from build123d import *

# Parameters (mm, degrees)
F0_R        = 15
F0_R_2      = 12
F1_DEPTH    = 1
F0_R_3      = 11.25
F2_DEPTH    = 7
F3_START    = 5
F1_FACE_R   = 15
F1_FACE_R_2 = 12
F3_DEPTH    = 1
F4_R        = 2


with BuildPart() as f1:
    # F0 (on Top) → F1 (new body)
    with BuildSketch(Plane.XY):
        Circle(F0_R)
        Circle(F0_R_2, mode=Mode.SUBTRACT)
    extrude(amount=F1_DEPTH)

    # F0 (on Top) → F2 (join)
    with BuildSketch(Plane.XY):
        Circle(F0_R_2)
        Circle(F0_R_3, mode=Mode.SUBTRACT)
    extrude(amount=F2_DEPTH)

    # F1_face (on face) → F3 (join)
    with BuildSketch(Plane.XY.offset(1).offset(F3_START)):
        Circle(F1_FACE_R)
        Circle(F1_FACE_R_2, mode=Mode.SUBTRACT)
    extrude(amount=F3_DEPTH)

    # F4
    f4_edges = [f1.edges().sort_by_distance(p)[0] for p in [
        (12, 0, 3.5),
        (-12, 0, 6),
        (-12, 0, 1),
    ]]
    fillet(f4_edges, radius=F4_R)


solid = f1.part
Check sheet for the modelled part. Datum: model origin and axes. Units: mm. Give positions to 0.01 mm unless a question says otherwise; leave off trailing zeros. Write each loop counter-clockwise with the first axis right and the second up, starting at its lowest first coordinate (ties: lowest second). Pieces come first, ordered by that corner, then holes. Notation, with made-up numbers: M 23,57 L 70,57 A20 cw 70,73 Z; hole C 41.25,-0.75 d8. An arc over 180 degrees is marked long. Use one line per item in the form item = value.
(1) Section check D-D on z = 5. Record the boundary of the cut face in (x, y), plus the area to 3 significant figures.
Answer block:
outline = C 0,0 d24.54; hole C 0,0 d22.5
area = 75.2 mm2
(2) Section check C-C on z = 2.5. Record the boundary of the cut face in (x, y), plus the area to 3 significant figures.
Answer block:
outline = C 0,0 d24.13; hole C 0,0 d22.5
area = 59.6 mm2
(3) Material ranges on line 1 along Y through (x, z) = (0, 3); line 2 along Z through (x, y) = (-11.5, -7.25); line 3 along X through (y, z) = (8.25, 5.75), recorded low to high.
Answer block:
line_1 = -12 to -11.25, 11.25 to 12
line_2 = 0 to 1.04, 5.96 to 7
line_3 = -10.09 to -7.65, 7.65 to 10.09
(4) Depth check by flat-ended pin: P1, Ø8, axis at x = 2.5, y = 3, coming from the +Z side; P2, Ø1, axis at x = 7, z = 2, coming from the +Y side. Enter the tip coordinate at first touch or a pass-through.
Answer block:
P1 = through
P2 = 10.65
(5) Section check A-A on y = 0. Record the boundary of the cut face in (x, z).
Answer block:
outline = M -15,0 L -11.25,0 L -11.25,7 L -15,7 L -15,6 L -14,6 A2 cw -12,4 L -12,3 A2 cw -14,1 L -15,1 Z; M 11.25,0 L 15,0 L 15,1 L 14,1 A2 cw 12,3 L 12,4 A2 cw 14,6 L 15,6 L 15,7 L 11.25,7 Z
(6) Draft check along Z on faces 1 (the flat face through (2.2, 11.2, 0)), 2 (the flat face through (2.2, 11.2, 7)), 3 (the cylindrical face through (-11.99, 0.53, 3.49)), 4 (the cylindrical face through (-14.985, 0.66, 6.493)). Enter one of: pulls with the +Z half, pulls with the -Z half, needs draft (parallel to the pull), parting line crosses it, or undercut.
Answer block:
face_1 = pulls with the -Z half
face_2 = pulls with the +Z half
face_3 = undercut
face_4 = needs draft
